from build123d import *

# Parameters (mm, degrees)
SKETCH1_W               = 60
SKETCH1_H               = 35
BOSS_EXTRUDE1_DEPTH     = 13
CUT_EXTRUDE1_DEPTH      = 64.837684937
CUT_EXTRUDE1_DEPTH_BACK = 64.837684937
SKETCH3_R               = 1.75
SKETCH5_R               = 1.75
CUT_EXTRUDE3_DEPTH      = 38.08436341
CHAMFER1_SIZE           = 3
CUT_EXTRUDE4_DEPTH      = 7
CHAMFER2_SIZE           = 0.5


with BuildPart() as part:
    # Sketch1 → Boss-Extrude1 (new body)
    with BuildSketch(Plane.XY):
        Rectangle(SKETCH1_W, SKETCH1_H)
    extrude(amount=BOSS_EXTRUDE1_DEPTH)

    # Sketch2 → Cut-Revolve1 (revolve, cut)
    with BuildSketch(Plane.XY.offset(13)):
        with BuildLine():
            Line((-25, 0), (-25, 8.218127455))
            ThreePointArc((-25, 8.218127455), (-24.486963528, 9.469250598), (-23.243251097, 10))
            ThreePointArc((-23.243251097, 10), (-15.040879193, 9.611248064), (-6.94833646, 8.218127455))
            ThreePointArc((-6.94833646, 8.218127455), (0, 7.408356031), (6.94833646, 8.218127455))
            ThreePointArc((6.94833646, 8.218127455), (15.040879193, 9.611248064), (23.243251097, 10))
            ThreePointArc((23.243251097, 10), (24.486963528, 9.469250598), (25, 8.218127455))
            Line((25, 8.218127455), (25, 0))
            Line((25, 0), (-25, 0))
        make_face()
    revolve(axis=Axis((25, 0, 13), (-1, 0, 0)), mode=Mode.SUBTRACT)

    # Sketch3 → Cut-Extrude1 (cut, two sides: drawn at the far end of the back side and taken through both)
    with BuildSketch(Plane(origin=(30, 0, 0), x_dir=(0, 0, -1), z_dir=(1, 0, 0)).offset(-CUT_EXTRUDE1_DEPTH_BACK)):
        with Locations((-13, 0)):
            Circle(SKETCH3_R)
    extrude(amount=CUT_EXTRUDE1_DEPTH + CUT_EXTRUDE1_DEPTH_BACK, mode=Mode.SUBTRACT)

    # Sketch5 → Cut-Extrude3 (cut, through all)
    with BuildSketch(Plane.XY.offset(13)):
        with Locations((0, 11.25)):
            Circle(SKETCH5_R)
        with Locations((0, -11.25)):
            Circle(SKETCH5_R)
    extrude(amount=-CUT_EXTRUDE3_DEPTH, mode=Mode.SUBTRACT)

    # Chamfer1
    chamfer1_edges = [part.edges().sort_by_distance(p)[0] for p in [
        (-30, 0, 0),
        (30, 0, 0),
    ]]
    chamfer(chamfer1_edges, length=CHAMFER1_SIZE)

    # Sketch6 → Cut-Extrude4 (cut)
    with BuildSketch(Plane(origin=(0, 0, 0), x_dir=(-1, 0, 0), z_dir=(0, 0, -1))):
        Polygon((3.464101615, 11.25), (1.732050808, 14.25), (-1.732050808, 14.25), (-3.464101615, 11.25), (-1.732050808, 8.25), (1.732050808, 8.25), align=None)
        Polygon((3.464101615, -11.25), (1.732050808, -8.25), (-1.732050808, -8.25), (-3.464101615, -11.25), (-1.732050808, -14.25), (1.732050808, -14.25), align=None)
    extrude(amount=-CUT_EXTRUDE4_DEPTH, mode=Mode.SUBTRACT)

    # Chamfer2
    chamfer2_edges = [part.edges().sort_by_distance(p)[0] for p in [
        (-2.598076211, 9.75, 0),
        (-2.598076211, 12.75, 0),
        (0, 14.25, 0),
        (2.598076211, 12.75, 0),
        (2.598076211, 9.75, 0),
        (0, 8.25, 0),
        (-2.598076211, 9.75, 7),
        (0, 8.25, 7),
        (2.598076211, 9.75, 7),
        (2.598076211, 12.75, 7),
        (0, 14.25, 7),
        (-2.598076211, 12.75, 7),
        (-1.75, 11.25, 7),
        (-2.598076211, -12.75, 0),
        (-2.598076211, -9.75, 0),
        (0, -8.25, 0),
        (2.598076211, -9.75, 0),
        (2.598076211, -12.75, 0),
        (0, -14.25, 0),
        (-2.598076211, -12.75, 7),
        (0, -14.25, 7),
        (2.598076211, -12.75, 7),
        (2.598076211, -9.75, 7),
        (0, -8.25, 7),
        (-2.598076211, -9.75, 7),
        (-1.75, -11.25, 7),
    ]]
    chamfer(chamfer2_edges, length=CHAMFER2_SIZE)


solid = part.part
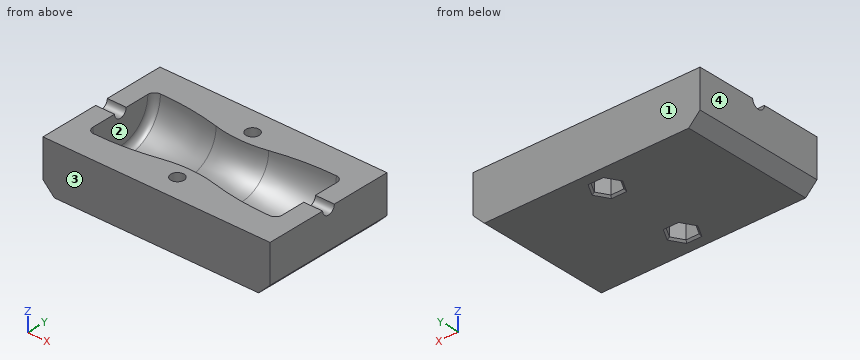
CAD build for the part. Positions are in the model's coordinates, mm. Face numbers are marked on the shaded views. Round coordinates to 2 decimals unless told otherwise and drop trailing zeros. Write each loop counter-clockwise with the first axis right and the second up, starting at its lowest first coordinate (ties: lowest second). Pieces come first, ordered by that corner, then holes. Notation, with made-up numbers: M 63.25,82.25 L 99.25,82.25 A17 cw 99.25,90.25 Z; hole C 15,81 d3. An arc over 180 degrees is marked long. Put each result on its own line as item: value. Start each with the question number.
1) Saw through at D-D, the plane x = -24. Write the cut outline in (y, z).
2) Pin check, flat tips, straight feed: pin 1 Ø5.5 at (x, y) = (0.5, -11) entering from -Z; pin 2 Ø5 at (x, y) = (11, -0.5) entering from +Z; pin 3 Ø5.5 at (x, y) = (0, 11.25) entering from -Z. Stop position of each tip, or through.
3) Drill centre lines: probe 1 along Y at (x, z) = (0, 11.1); probe 2 along Y at (x, z) = (0, 9.75); probe 3 along X at (y, z) = (2.5, 10.25). Where is each one in solid material? Low to high. Write a range as [from, to].
4) Pull direction Y, two halves, no side cores. Call the marked faces 1, 2, 3 and 4: pulls with the +Y half, pulls with the -Y half, needs draft (parallel to the pull), parting line crosses it, or undercut.
5) Saw through at A-A, the plane z = 2. Write the cut outline in (x, y), and give its area (3 significant figures).
6) Saw through at B-B, the plane x = 0. Count the separate pieces of the cut face and the enclosed holes in it, and give its area (3 significant figures).
Resolved:
1. outline: M -17.5,0 L 17.5,0 L 17.5,13 L 9.82,13 A9.82 cw -9.82,13 L -17.5,13 Z
2. pin 1: z = 0.19
2. pin 2: z = 4.6
2. pin 3: z = 6.75
3. probe 1: [-17.5, -13], [-9.5, -7.16], [7.16, 9.5], [13, 17.5]
3. probe 2: [-17.5, -13], [-9.5, -6.66], [6.66, 9.5], [13, 17.5]
3. probe 3: [-30, -25], [25, 30]
4. face 1: pulls with the +Y half
4. face 2: undercut
4. face 3: pulls with the -Y half
4. face 4: needs draft
5. outline: M -29,-17.5 L 29,-17.5 L 29,17.5 L -29,17.5 Z; hole M -3.46,-11.25 L -1.73,-14.25 L 1.73,-14.25 L 3.46,-11.25 L 1.73,-8.25 L -1.73,-8.25 Z; hole M -3.46,11.25 L -1.73,8.25 L 1.73,8.25 L 3.46,11.25 L 1.73,14.25 L -1.73,14.25 Z
5. area: 1,970 mm²
6. separate pieces: 3
6. enclosed holes: 0
6. area: 242 mm²
